Autodesk Inventor part; units mm, degrees
ref_plane "YZ Plane" through (0, 0, 0) normal (1, 0, 0) x (0, 1, 0)
ref_plane "XZ Plane" through (0, 0, 0) normal (0, 1, 0) x (-1, 0, 0)
ref_plane "XY Plane" through (0, 0, 0) normal (0, 0, 1) x (1, 0, 0)
sketch "Sketch1" plane through (0, 0, 0) normal (0, 0, 1) x (1, 0, 0)
  line L0 (-914.4, 0) -> (914.4, 0)
  line L1 (-914.4, 2482.85) -> (-914.4, -2393.95)
  line L2 (914.4, -2393.95) -> (914.4, 2482.85)
  line L3 (-914.4, -1155.7) -> (914.4, -1155.7)
  line L4 (914.4, -52.5818) -> (-831.1936, -1155.7)
  line L5 (-914.4, -1103.1182) -> (831.1936, 0)
  line L6 (914.4, -52.5818) -> (914.4, 0)
  line L7 (914.4, 0) -> (831.1936, 0)
  line L8 (-914.4, -1103.1182) -> (-914.4, -1155.7)
  line L9 (-831.1936, -1155.7) -> (-914.4, -1155.7)
  point P0 (0, 0)
extrude "Extrusion1" add sketch "Sketch1" against normal blind 38.1 contours L0 L2 L4 L3 L1 L5
properties part number "side2"
Input: part model. Units: mm. Frame: model coordinates. Coordinates: 2 decimals unless noted, no trailing zeros. Loops run counter-clockwise (first coordinate to the right, second up) from the corner with the lowest first, then second, coordinate; pieces in that order, holes last.
(1) First-contact query: pin 1 Ø10 at (x, z) = (582, -14) entering from +Y; pin 2 Ø8 at (y, z) = (-937, -10.5) entering from +X; pin 3 Ø1 at (x, z) = (84, -22.5) entering from -Y. Flat tips, straight axial feed; report the tip coordinate or a pass-through.
(2) Section A-A on z = -21.5. Return the cut outline in (x, y).
(3) Section B-B on x = -114. Return the cut outline in (y, z), then the cut area to 3 significant figures.
(4) Section C-C on y = -907. Return the cut outline in (x, z), then the cut area to 3 significant figures.
(5) Material intervals for probe 1 along Y at (x, z) = (-304, -16); probe 2 along Y at (x, z) = (-732.5, -11); probe 3 along X at (y, z) = (-973.5, -4.5), sorted ascending.
Data:
1. pin 1: stops at y = -154.32
1. pin 2: stops at x = -478.79
1. pin 3: stops at y = -577.66
2. outline: (-914.4, -1155.7) - (-831.19, -1155.7) - (914.4, -52.58) - (914.4, 0) - (831.19, 0) - (-914.4, -1103.12) - close
3. outline: (-702.47, -38.1) - (-597.31, -38.1) - (-597.31, 0) - (-702.47, 0) - close
3. area: 4,010 mm2
4. outline: (-604.06, -38.1) - (-437.65, -38.1) - (-437.65, 0) - (-604.06, 0) - close
4. area: 6,340 mm2
5. probe 1: y = -822.54 to -717.38
5. probe 2: y = -1093.33 to -988.17
5. probe 3: x = -709.29 to -542.88
